Check sheet for the modelled part. Datum: model origin and axes. Units: mm. A direction names the side the tool comes from. Round coordinates to 2 decimals unless told otherwise and drop trailing zeros. Write each loop counter-clockwise with the first axis right and the second up, starting at its lowest first coordinate (ties: lowest second). Pieces come first, ordered by that corner, then holes. Notation, with made-up numbers: (71, 58.5) - (124, 58.5) arc R22 ccw to (124, 75.5) - close; hole circle Ø8 at (-19.75, 78.5). An arc over 180 degrees is marked (long way). Answer as a JSON object with one key per item and string values. Group by question number.
Item 1: Sectioned sample at B-B on z = 211.5. Record the boundary of the cut face in (x, y).
Item 2: Gauge pin test, flat end, axial feed: P1, Ø8, axis at y = -133.5, z = 348.5, coming from the +X side. Record the tip position at first contact, or that the pin passes through.
Item 3: Set-up check for faces 1 (the flat face through (477.774, -245.545, 175.311)), 2 (the flat face through (445, -107, 355.6)), 3 (the flat face through (1906, -107, 355.6)): record each of +Z, -Z, +X, -X, +Y, -Y from which the full face is reachable in a straight line by a thin tool's end or side.
Item 4: Sectioned sample at C-C on x = 1665. Record the boundary of the cut face in (y, z).
Item 5: Thickness scan on line 1 (Z direction, x = 551, y = -48.5); line 2 (Z direction, x = 1096, y = -250); line 3 (X direction, y = -110, z = 353.5). Record the ranges inside material, lowest first.
```python
from build123d import *

# Parameters (mm, degrees)
F1_DEPTH = 355.6
F2_W     = 635
F2_H     = 279.345146747
F3_DEPTH = 38.1
F4_SIZE  = 38.09999
F5_SIZE  = 38.1


# Not quite as in the source:
# - a fillet or chamfer is up to 0.001 mm smaller than in the source, because OpenCascade refuses the exact size


with BuildPart() as f1:
    # F0 (on Top) → F1 (new body)
    with BuildSketch(Plane.XY):
        Polygon((2363.263666194, 0), (0, 0), (0, -127), (102.108, -212.6787851403), (864.108, -279.345146747), (1499.108, -279.345146747), (2261.108, -212.7113899342), (2363.263666194, -127), align=None)
    extrude(amount=F1_DEPTH)

    # F2 (on face) → F3 (join)
    with BuildSketch(Plane.XY.offset(355.6)):
        with Locations((1181.608, -139.6725733735)):
            Rectangle(F2_W, F2_H)
    extrude(amount=F3_DEPTH)

    # F4 (size 38.1 in the source; OpenCascade refuses exactly that, so slightly less here)
    f4_edges = [f1.edges().sort_by_distance(p)[0] for p in [
        (864.108, -139.672573, 393.7),
        (1499.108, -139.672573, 393.7),
    ]]
    chamfer(f4_edges, length=F4_SIZE)

    # F5
    f5_edges = [f1.edges().sort_by_distance(p)[0] for p in [
        (0, -63.5, 355.6),
        (1181.608, -279.345147, 393.7),
        (2363.263666, -63.5, 355.6),
    ]]
    chamfer(f5_edges, length=F5_SIZE)


solid = f1.part
```
Completed:
{
 "1": {"outline": "(0, -127) - (102.11, -212.68) - (864.11, -279.35) - (1499.11, -279.35) - (2261.11, -212.71) - (2363.26, -127) - (2363.26, 0) - (0, 0) - close"},
 "2": {"P1": "x = 2336.26"},
 "3": {"face 1": "+Z, -Z, -X, -Y", "face 2": "+Z, -X, +Y, -Y", "face 3": "+Z, +X, +Y, -Y"},
 "4": {"outline": "(-264.84, 0) - (0, 0) - (0, 355.6) - (-264.84, 355.6) - close"},
 "5": {"line 1": "0 to 355.6", "line 2": "0 to 384.95", "line 3": "36 to 2327.26"}
}
